```python
from build123d import *

# Parameters (mm, degrees)
MODEL_R             = 1.500000002
MODEL_R_2           = 1.300000002
MODEL_R_3           = 1.500000003
MODEL_W             = 3
MODEL_H             = 6
MODEL_W_2           = 10
MODEL_H_2           = 3
MODEL_W_3           = 23
MODEL_H_3           = 12
BOSS_EXTRUDE1_DEPTH = 3


with BuildPart() as part:
    # Model → Boss-Extrude1 (new body)
    with BuildSketch(Plane.XY):
        with BuildLine():
            Line((28.47306014, 22.66800001), (28.473164499, 63.3680236))
            ThreePointArc((28.473164499, 63.3680236), (29.351812484, 65.489297995), (31.473064499, 66.36800001))
            Line((31.473064499, 66.36800001), (85.473064499, 66.36800001))
            ThreePointArc((85.473064499, 66.36800001), (87.594368353, 65.489496156), (88.473064511, 63.368271953))
            Line((88.473064511, 63.368271953), (88.473064511, 22.66800001))
            ThreePointArc((88.473064511, 22.66800001), (87.594512967, 20.546548464), (85.47306014, 19.66800001))
            Line((85.47306014, 19.66800001), (31.47306014, 19.66800001))
            ThreePointArc((31.47306014, 19.66800001), (29.351710139, 20.54665001), (28.47306014, 22.66800001))
        make_face()
        with Locations((32.973060142, 32.168000012)):
            Circle(MODEL_R, mode=Mode.SUBTRACT)
        with Locations((58.473060142, 60.168000012)):
            Circle(MODEL_R, mode=Mode.SUBTRACT)
        with Locations((67.973060142, 22.668000012)):
            Circle(MODEL_R_2, mode=Mode.SUBTRACT)
        with Locations((67.973060142, 40.668000012)):
            Circle(MODEL_R_2, mode=Mode.SUBTRACT)
        with Locations((83.97306014, 52.16800001)):
            Circle(MODEL_R_3, mode=Mode.SUBTRACT)
        with Locations((32.97306014, 38.66800001)):
            Rectangle(MODEL_W, MODEL_H, mode=Mode.SUBTRACT)
        with Locations((40.97306014, 60.16800001)):
            Rectangle(MODEL_W_2, MODEL_H_2, mode=Mode.SUBTRACT)
        with Locations((32.97306014, 25.66800001)):
            Rectangle(MODEL_W, MODEL_H, mode=Mode.SUBTRACT)
        with Locations((75.97306014, 60.16800001)):
            Rectangle(MODEL_W_2, MODEL_H_2, mode=Mode.SUBTRACT)
        with Locations((83.97306014, 58.66800001)):
            Rectangle(MODEL_W, MODEL_H, mode=Mode.SUBTRACT)
        with Locations((83.97306014, 45.66800001)):
            Rectangle(MODEL_W, MODEL_H, mode=Mode.SUBTRACT)
        with Locations((67.97306014, 31.66800001)):
            Rectangle(MODEL_W_3, MODEL_H_3, mode=Mode.SUBTRACT)
    extrude(amount=BOSS_EXTRUDE1_DEPTH)


solid = part.part
```
Verification items for the finished model (mm, model axes). A direction names the side the tool comes from. Coordinates: 2 decimals unless noted, no trailing zeros. Order: outer loops, then holes, each group sorted by start corner. A loop starts at its lowest first (then second) coordinate and runs counter-clockwise, first axis right, second up. Notation, with made-up numbers: (88, -13) -> (120, -13) arc R26 cw to (120, 9) -> close; hole circle Ø1 at (2, 79). An arc over 180 degrees is marked (long way). Put each result on its own line as item: value. Start each with the question number.
1) Cross-section at D-D (y = 46.5). Enter the section's corners in (x, z), plus the area to 3 significant figures.
2) Tool access check on faces 1 (the flat face through (70.973, 60, 1)), 2 (the cylindrical face through (29.33, 65.47, 1.48)). Record the directions out of +Z, -Z, +X, -X, +Y, -Y that give a thin tool (end or side, any length) a straight path to the whole face; none if there is none.
3) Release check for a two-part mould opening along Y. For faces 3 (the flat face through (59, 19.668, 1)), 4 (the cylindrical face through (57.28, 59.26, 1.48)), 5 (the flat face through (59, 43, 0)) record: pulls with the +Y half, pulls with the -Y half, needs draft (parallel to the pull), parting line crosses it, or undercut.
4) Material ranges on L1, parallel to Y at x = 74, z = 1.65; L2, parallel to X at y = 32, z = 1.35; L3, parallel to X at y = 46, z = 0.2, recorded low to high.
5) Cross-section at B-B (x = 72.5). Enter the section's corners in (y, z), plus the area to 3 significant figures.
6) Cross-section at A-A (x = 65). Enter the section's corners in (y, z), plus the area to 3 significant figures.
7) Cross-section at C-C (y = 27.5). Enter the section's corners in (x, z), plus the area to 3 significant figures.
Geometry check:
1. outline: (28.47, 0) -> (82.47, 0) -> (82.47, 3) -> (28.47, 3) -> close; (85.47, 0) -> (88.47, 0) -> (88.47, 3) -> (85.47, 3) -> close
1. area: 171 mm^2
2. face 1: +Z, -Z
2. face 2: +Z, -Z, -X, +Y
3. face 3: pulls with the -Y half
3. face 4: undercut
3. face 5: needs draft
4. L1: y = 19.67 to 25.67, 37.67 to 58.67, 61.67 to 66.37
4. L2: x = 28.47 to 31.48, 34.46 to 56.47, 79.47 to 88.47
4. L3: x = 28.47 to 82.47, 85.47 to 88.47
5. outline: (19.67, 0) -> (25.67, 0) -> (25.67, 3) -> (19.67, 3) -> close; (37.67, 0) -> (58.67, 0) -> (58.67, 3) -> (37.67, 3) -> close; (61.67, 0) -> (66.37, 0) -> (66.37, 3) -> (61.67, 3) -> close
5. area: 95.1 mm^2
6. outline: (19.67, 0) -> (25.67, 0) -> (25.67, 3) -> (19.67, 3) -> close; (37.67, 0) -> (66.37, 0) -> (66.37, 3) -> (37.67, 3) -> close
6. area: 104 mm^2
7. outline: (28.47, 0) -> (31.47, 0) -> (31.47, 3) -> (28.47, 3) -> close; (34.47, 0) -> (56.47, 0) -> (56.47, 3) -> (34.47, 3) -> close; (79.47, 0) -> (88.47, 0) -> (88.47, 3) -> (79.47, 3) -> close
7. area: 102 mm^2
